from build123d import *

# Parameters (mm, degrees)
BOSS_EXTRUDE1_DEPTH      = 15
BOSS_EXTRUDE1_DEPTH_BACK = 15
SKETCH1_R                = 125
SKETCH2_R                = 25
BOSS_EXTRUDE2_DEPTH      = 20
SKETCH3_R                = 2.5
BOSS_EXTRUDE3_DEPTH      = 15
CIRPATTERN1_COUNT        = 4
BOSS_EXTRUDE4_DEPTH      = 10


with BuildPart() as part:
    # Sketch1 → Boss-Extrude1 (new, two sides: drawn at the far end of the back side and taken through both)
    with BuildSketch(Plane.XY.offset(-BOSS_EXTRUDE1_DEPTH_BACK)):
        with Locations((-0.2079628, -0.516116692)):
            Circle(SKETCH1_R)
        Polygon((-30, 430), (30, 430), (30, 30), (430, 30), (430, -30), (30, -30), (30, -430), (-30, -430), (-30, -30), (-430, -30), (-430, 30), (-30, 30), align=None)
    extrude(amount=BOSS_EXTRUDE1_DEPTH + BOSS_EXTRUDE1_DEPTH_BACK)

    # Sketch2 → Boss-Extrude2 (add)
    with BuildSketch(Plane.XY.offset(15)):
        with Locations((390, 0)):
            Circle(SKETCH2_R)
    boss_extrude2 = extrude(amount=BOSS_EXTRUDE2_DEPTH)

    # Sketch3 → Boss-Extrude3 (add)
    with BuildSketch(Plane.XY.offset(35)):
        with Locations((390, 0)):
            Circle(SKETCH3_R)
    boss_extrude3 = extrude(amount=BOSS_EXTRUDE3_DEPTH)

    # CirPattern1: Boss-Extrude2, Boss-Extrude3 ×4 about axis
    cirpattern1_axis = Axis((-0.2079628, -0.516116692, 0), (0, 0, 1))
    add([boss_extrude2.rotate(cirpattern1_axis, i * 360 / CIRPATTERN1_COUNT) for i in range(1, CIRPATTERN1_COUNT)])
    add([boss_extrude3.rotate(cirpattern1_axis, i * 360 / CIRPATTERN1_COUNT) for i in range(1, CIRPATTERN1_COUNT)])

    # Sketch4 → Boss-Extrude4 (add)
    with BuildSketch(Plane.XY.offset(15)):
        Polygon((-5.834664758, -5.834664758), (67.788123176, -79.457452693), (79.457452693, -67.788123176), (5.834664758, 5.834664758), align=None)
    extrude(amount=BOSS_EXTRUDE4_DEPTH)


solid = part.part
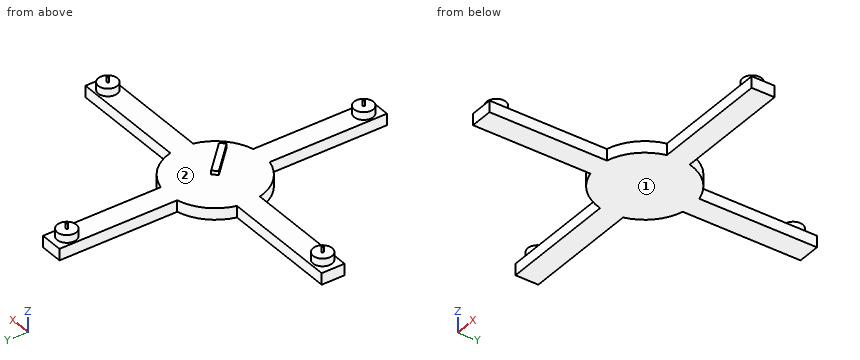
Can you work these out from the model? Positions are in its coordinate system, mm. Face numbers are marked on the shaded views. Coordinates: 2 decimals unless noted, no trailing zeros. Loops run counter-clockwise (first coordinate to the right, second up) from the corner with the lowest first, then second, coordinate; pieces in that order, holes last. Notation, with made-up numbers: (-4, 81.25) - (2, 81.25) arc R11 cw to (2, 102.25) - close; hole circle Ø10 at (79, 44.25). An arc over 180 degrees is marked (long way). Answer as a JSON object with one key per item and string values. Group by question number.
Item 1: If we section it at B-B (y = 237): List the corners of the cut face in (x, z) for me.
Item 2: If I drill on L1, parallel to Z at x = 101, y = 51; L2, parallel to Y at x = 263, z = -6, over which ranges is the centre line in solid material (lowest first)? Write a range as from..to.
Item 3: For pin 1 (15 mm diameter, centred on y = -338.5, z = 2, fed in from +X); pin 2 (10 mm diameter, centred on y = 155, z = 2.5, fed in from -X); pin 3 (24 mm diameter, centred on x = 313.5, z = 7, fed in from -Y); pin 4 (25 mm diameter, centred on x = 11, y = 399, fed in from +Z), each with a flat end and sliding along its axis, tell me the tip position at first contact or that it passes through.
Item 4: If we section it at A-A (z = 0): List the corners of the cut face in (x, y) for me.
Item 5: If we mould it in two halves opening along X, with no side actions, what happens to the marked faces 1 and 2? For each: released by +X, released by -X, zero draft, split by the parting line, or undercut.
Returned:
{
 "1": {"outline": "(-30, -15) - (30, -15) - (30, 15) - (-30, 15) - close"},
 "2": {"L1": "z = -15..15", "L2": "y = -30..30"},
 "3": {"pin 1": "stops at x = 30", "pin 2": "stops at x = -30", "pin 3": "stops at y = -30", "pin 4": "stops at z = 50"},
 "4": {"outline": "(-430, -30) - (-121.68, -30) arc R125 ccw to (-30, -121.91) - (-30, -430) - (30, -430) - (30, -121.81) arc R125 ccw to (121.27, -30) - (430, -30) - (430, 30) - (121.01, 30) arc R125 ccw to (30, 120.78) - (30, 430) - (-30, 430) - (-30, 120.88) arc R125 ccw to (-121.43, 30) - (-430, 30) - close"},
 "5": {"face 1": "zero draft", "face 2": "undercut"}
}
